For this review, use the dimensioned drawing (mm, ordinates from the lowest corner) and the shaded views. A direction names the side the tool comes from. Coordinates: 2 decimals unless noted, no trailing zeros. Write each loop counter-clockwise with the first axis right and the second up, starting at its lowest first coordinate (ties: lowest second). Pieces come first, ordered by that corner, then holes. Notation, with made-up numbers: M -7,88 L 41,88 A30 cw 41,118 Z; hole C 76,23.5 d9. An arc over 180 degrees is marked long. Return JSON: item names as keys, results as strings.
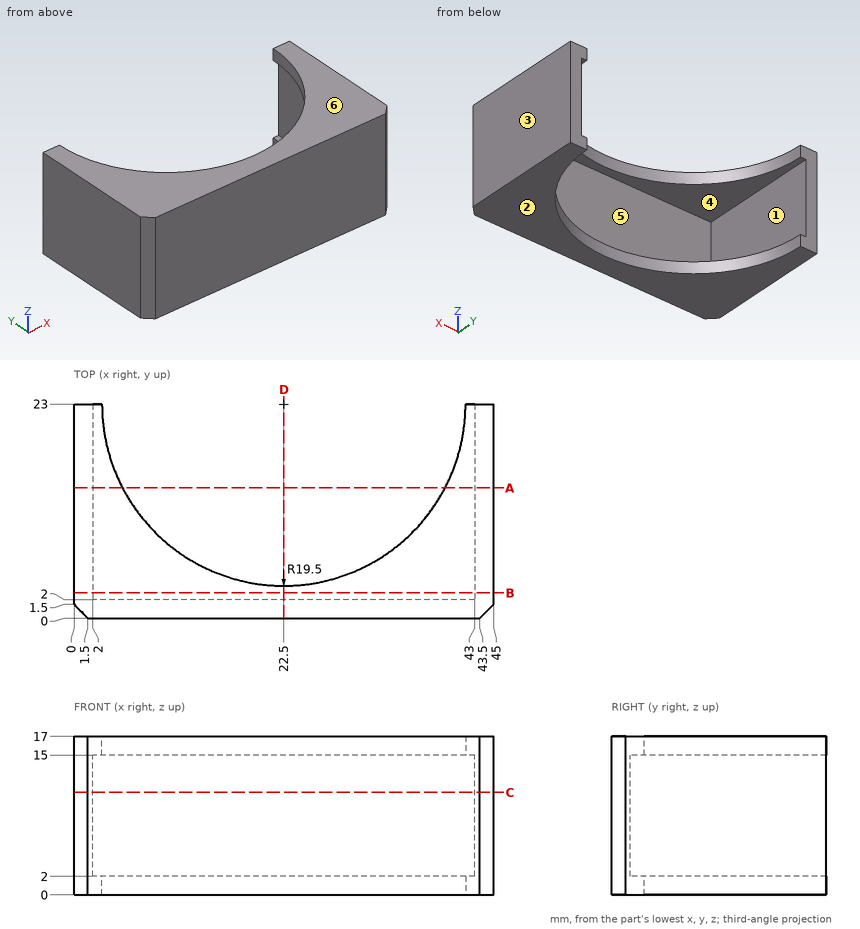
1. Wall thickness on L1, parallel to Z at x = 4, y = 7.75; L2, parallel to X at y = 21.25, z = 9.25; L3, parallel to Y at x = 15.5, z = 4.75: over which ranges is each line inside the solid? List them lowest first. Write a range as from..to.
Checks:
{"L1": "0..2, 15..17", "L2": "0..2, 43..45", "L3": "0..2"}
2. We need section A-A (y = 14). State the section outline as (x, z) points, plus the area to 3 significant figures.
Checks:
{"outline": "M 0,0 L 5.2,0 L 5.2,2 L 2,2 L 2,15 L 5.2,15 L 5.2,17 L 0,17 Z; M 39.8,0 L 45,0 L 45,17 L 39.8,17 L 39.8,15 L 43,15 L 43,2 L 39.8,2 Z", "area": "93.6 mm2"}
3. For the marked faces 5 and 6, list the 3-axis set-ups (+Z, -Z, +X, -X, +Y, -Y) from which the entire face can be reached by the end or side of a thin tool; tool diameter is ignored.
Checks:
{"face 5": "+Y", "face 6": "+Z, +X, -X, +Y, -Y"}
4. We need section D-D (x = 22.5). State the section outline as (y, z) points.
Checks:
{"outline": "M 0,0 L 3.5,0 L 3.5,2 L 2,2 L 2,15 L 3.5,15 L 3.5,17 L 0,17 Z"}
5. We need section B-B (y = 2.75). State the section outline as (x, z) points, plus the area to 3 significant figures.
Checks:
{"outline": "M 0,0 L 45,0 L 45,17 L 0,17 Z; hole M 2,2 L 43,2 L 43,15 L 2,15 Z", "area": "232 mm2"}
6. Draft analysis for pull direction X (two halves, no side actions). For the marked faces 1, 2, 3 and 4, state which applies: +X half, -X half, draft (parallel to the pull), parting line (faces both ways), or undercut.
Checks:
{"face 1": "undercut", "face 2": "draft", "face 3": "+X half", "face 4": "undercut"}
7. We need section C-C (z = 11). State the section outline as (x, y) points.
Checks:
{"outline": "M 0,1.5 L 1.5,0 L 43.5,0 L 45,1.5 L 45,23 L 43,23 L 43,2 L 2,2 L 2,23 L 0,23 Z"}
8. Clearance check with flat-ended pins moving along their axes: pin 1 Ø1.5 at (y, z) = (17.5, 15) entering from -X; pin 2 Ø10 at (x, z) = (16.5, 7.5) entering from +Y; pin 3 Ø10.5 at (x, y) = (23, 11.5) entering from -Z. State where each tip first meets the part, or that it passes through.
Checks:
{"pin 1": "x = 0", "pin 2": "y = 2", "pin 3": "through"}
